Autodesk Inventor part; units mm, degrees
ref_plane "YZ Plane" through (0, 0, 0) normal (1, 0, 0) x (0, 1, 0)
ref_plane "XZ Plane" through (0, 0, 0) normal (0, 1, 0) x (-1, 0, 0)
ref_plane "XY Plane" through (0, 0, 0) normal (0, 0, 1) x (1, 0, 0)
sketch "Sketch1" plane through (0, 0, 0) normal (1, 0, 0) x (0, 1, 0)
  line L0 (0, 0) -> (12.5, 0)
  line L1 (12.5, 0) -> (12.5, -5)
  line L2 (12.5, -5) -> (0, -5)
  line L3 (0, 0) -> (0, 5)
  line L4 (0, 5) -> (15, 5)
  line L5 (15, 5) -> (15, -10)
  line L6 (15, -10) -> (0, -10)
  line L7 (0, -10) -> (0, -5)
  dimension "d0" = 12.5
  dimension "d2" = 5
  dimension "d3" = 15
  dimension "d4" = 15
  dimension "d5" = 5
extrude "Extrusion1" add sketch "Sketch1" along normal blind 27.5
sketch "Sketch2" plane through (0, 0, 5) normal (0, 0, 1) x (1, 0, 0)
  line L0 (0, 15) -> (27.5, 15)
  line L1 (0, 15) -> (0, 36)
  line L2 (0, 36) -> (2.5, 36)
  line L3 (0, 15) -> (39.5, 15)
  line L4 (39.5, 15) -> (39.5, 36)
  line L5 (39.5, 36) -> (37, 36)
  line L6 (37, 36) -> (37, 17.5)
  line L7 (37, 17.5) -> (2.5, 17.5)
  line L8 (2.5, 17.5) -> (2.5, 36)
  line L9 (0, 0) -> (27.5, 0)
  dimension "d8" = 21
  dimension "d9" = 2.5
  dimension "d10" = 39.5
  dimension "d11" = 2.5
  dimension "d12" = 18.5
  dimension "d13" = 17.5
extrude "Extrusion2" add sketch "Sketch2" against normal up to surface (15 mm away)
sketch "Sketch3" plane through (27.5, 0, -10) normal (0, 0, -1) x (-1, 0, 0)
  line L0 (27.5, 0) -> (22, 0)
  line L1 (22, 0) -> (22, 15)
  line L2 (22, 15) -> (27.5, 15)
  line L3 (27.5, 15) -> (27.5, 0)
  dimension "d16" = 5.5
  dimension "d17" = 15
extrude "Extrusion3" cut sketch "Sketch3" against normal up to surface (15 mm away)
sketch "Sketch4" plane through (37, 17.5, -10) normal (0, 0, -1) x (-1, 0, 0)
  line L0 (-2.5, -2.5) -> (9.5, -2.5)
  line L1 (37, 18.5) -> (34.5, 18.5)
  line L2 (-2.5, -2.5) -> (37, -2.5)
  line L3 (37, -2.5) -> (37, 18.5)
  line L4 (37, 18.5) -> (-2.5, 18.5)
  line L5 (-2.5, 18.5) -> (-2.5, -2.5)
  point P0 (37, -17.5)
extrude "Extrusion4" add sketch "Sketch4" along normal blind 2.5
sketch "Sketch5" plane through (2.5, 17.5, 5) normal (0, 0, 1) x (1, 0, 0)
  line L0 (37, -2.5) -> (25, -2.5)
  line L1 (37, 18.5) -> (37, -2.5)
  line L2 (34.5, 18.5) -> (37, 18.5)
  line L3 (34.5, 0) -> (34.5, 18.5)
  line L4 (0, 0) -> (34.5, 0)
  line L5 (0, 18.5) -> (0, 0)
  line L6 (-2.5, 18.5) -> (0, 18.5)
  line L7 (-2.5, -2.5) -> (-2.5, 18.5)
  line L8 (-2.5, -2.5) -> (3, -2.5)
  line L9 (37, 18.5) -> (37, -2.5)
  line L10 (37, -2.5) -> (25, -2.5)
  line L11 (37, 18.5) -> (34.5, 18.5)
  line L12 (34.5, 18.5) -> (34.5, 0)
  line L13 (34.5, -2.5) -> (37, -2.5)
  line L14 (37, -2.5) -> (37, 18.5)
  line L15 (0, 18.5) -> (0, 0)
  line L16 (-2.5, -2.5) -> (3, -2.5)
  line L17 (0, 18.5) -> (-2.5, 18.5)
  line L18 (-2.5, 18.5) -> (-2.5, -2.5)
  line L19 (-2.5, -2.5) -> (0, -2.5)
  line L20 (0, 0) -> (0, 18.5)
  line L21 (0, 0) -> (34.5, 0)
  line L22 (0, 0) -> (34.5, 0)
  line L23 (0, -2.5) -> (34.5, -2.5)
  line L24 (37, -2.5) -> (-2.5, -2.5)
  dimension "d22" = 34.5
  dimension "d23" = 34.5
extrude "Extrusion5" add sketch "Sketch5" along normal blind 2.5
sketch "Sketch6" plane through (2.5, 36, -10) normal (0, 1, 0) x (1, 0, 0)
  line L0 (37, -17.5) -> (37, 2.5)
  line L1 (-2.5, 2.5) -> (-2.5, -17.5)
  line L2 (37, 2.5) -> (-2.5, 2.5)
  line L3 (-2.5, 2.5) -> (-2.5, -17.5)
  line L4 (-2.5, -17.5) -> (37, -17.5)
  line L5 (37, -17.5) -> (37, 2.5)
  point P0 (-2.5, -10)
extrude "Extrusion6" add sketch "Sketch6" along normal blind 2.5
sketch "Sketch7" plane through (2.5, 17.5, 7.5) normal (0, 0, 1) x (1, 0, 0)
  line L0 (34.5, 18.5) -> (34.5, 0)
  line L1 (34.5, 0) -> (0, 0)
  line L2 (0, 0) -> (0, 18.5)
  line L3 (0, 18.5) -> (34.5, 18.5)
  line L4 (37, -2.5) -> (37, 21)
  line L5 (-2.5, 21) -> (37, 21)
  line L6 (-2.5, -2.5) -> (-2.5, 21)
  line L7 (-2.5, -2.5) -> (37, -2.5)
  line L8 (-2.5, -2.5) -> (37, -2.5)
  line L9 (37, 21) -> (34.5, 21)
  line L10 (34.5, 21) -> (34.5, -2.5)
  line L11 (34.5, -2.5) -> (37, -2.5)
  line L12 (37, -2.5) -> (37, 21)
  point P0 (-2.5, -17.5)
  dimension "d28" = 2.5
extrude "Extrusion7" cut sketch "Sketch7" against normal up to next contours L10 L5 L4 L7 L0
sketch "Sketch8" plane through (2.5, 17.5, 7.5) normal (0, 0, 1) x (1, 0, 0)
  line L0 (34.5, -2.5) -> (34.5, 0)
  line L1 (34.5, 0) -> (0, 0)
  line L2 (0, 0) -> (0, 18.5)
  line L3 (0, 18.5) -> (34.5, 18.5)
  line L4 (34.5, 18.5) -> (34.5, 21)
  line L5 (-2.5, 21) -> (34.5, 21)
  line L6 (-2.5, -2.5) -> (-2.5, 21)
  line L7 (-2.5, -2.5) -> (34.5, -2.5)
  line L8 (34.5, -2.5) -> (-2.5, -2.5)
  line L9 (-2.5, -2.5) -> (-2.5, 0)
  line L10 (0, 0) -> (34.5, 0)
  line L11 (34.5, 0) -> (34.5, -2.5)
  line L12 (34.5, 21) -> (-2.5, 21)
  line L13 (-2.5, 21) -> (-2.5, 18.5)
  line L14 (0, 18.5) -> (34.5, 18.5)
  line L15 (34.5, 18.5) -> (34.5, 21)
  line L16 (0, 18.5) -> (0, 0)
  line L17 (-2.5, 18.5) -> (-2.5, 0)
  dimension "d31" = 18.5
extrude "Extrusion8" add sketch "Sketch8" along normal blind 5
properties part number "battery-holder"
Can you work these out from the model? Positions are in its coordinate system, mm. A direction names the side the tool comes from. Coordinates: 2 decimals unless noted, no trailing zeros. Loops run counter-clockwise (first coordinate to the right, second up) from the corner with the lowest first, then second, coordinate; pieces in that order, holes last. Notation, with made-up numbers: (46.25, 62.25) - (60.25, 62.25) arc R12 cw to (60.25, 78.25) - close; hole circle Ø7 at (52, 85). An arc over 180 degrees is marked (long way). Answer as a JSON object with one key per item and string values. Group by question number.
Item 1: If we section it at A-A (y = 6.5): List the corners of the cut face in (x, z) for me, plus the area to 3 significant figures.
Item 2: If we section it at C-C (z = -7.75): List the corners of the cut face in (x, y) for me, plus the area to 3 significant figures.
Item 3: For pin 1 (6 mm diameter, centred on x = 25.5, z = -6, fed in from -Y); pin 2 (4.5 mm diameter, centred on x = 17, y = 4.5, fed in from +Z); pin 3 (1.5 mm diameter, centred on y = 23, z = -8, fed in from +X); pin 4 (6 mm diameter, centred on x = 21, y = 9, fed in from -Z), each with a flat end and sliding along its axis, tell me the tip position at first contact or that it passes through.
Item 4: If I drill on L1, parallel to Y at x = 26, z = -2; L2, parallel to Z at x = 18.5, y = 2; L3, parallel to Y at x = 6, z = 11.25, over which ranges is the centre line in solid material (lowest first)? Write a range as from..to.
Item 5: If we section it at D-D (y = 33): List the corners of the cut face in (x, z) for me.
Item 6: If we section it at B-B (x = 9.5): List the corners of the cut face in (y, z) for me, plus the area to 3 significant figures.
Item 7: On a 3-axis mill with a long thin cutter (end or side, diameter ignored), from which of +Z, -Z, +X, -X, +Y, -Y can I reach the whole of each face in a straight line? I mean faces 4 (the face through (16, 8, -10)), 5 (the face through (16, 6, -5)), 6 (the face through (5.5, 7, 1)), 7 (the face through (2.5, 27, 1)). Say none if no direction works.
Item 8: If we mould it in two halves opening along Z, with no side actions, what happens to faces 1 (the face through (16, 7, 5)), 2 (the face through (16, 6, 0)), 3 (the face through (20, 17.5, 1))? For each: released by +Z, released by -Z, zero draft, split by the parting line, or undercut.
Returned:
{
 "1": {"outline": "(5.5, -10) - (27.5, -10) - (27.5, -5) - (5.5, -5) - close; (5.5, 0) - (27.5, 0) - (27.5, 5) - (5.5, 5) - close", "area": "220 mm²"},
 "2": {"outline": "(0, 15) - (5.5, 15) - (5.5, 0) - (27.5, 0) - (27.5, 15) - (37, 15) - (37, 17.5) - (2.5, 17.5) - (2.5, 36) - (37, 36) - (37, 38.5) - (0, 38.5) - close", "area": "561 mm²"},
 "3": {"pin 1": "stops at y = 0", "pin 2": "stops at z = 5", "pin 3": "stops at x = 2.5", "pin 4": "stops at z = -10"},
 "4": {"L1": "y = 12.5..17.5, 36..38.5", "L2": "z = -10..-5, 0..5", "L3": "y = 15..17.5, 36..38.5"},
 "5": {"outline": "(0, -12.5) - (37, -12.5) - (37, -10) - (2.5, -10) - (2.5, 12.5) - (0, 12.5) - close"},
 "6": {"outline": "(0, -10) - (15, -10) - (15, -12.5) - (38.5, -12.5) - (38.5, 12.5) - (36, 12.5) - (36, -10) - (17.5, -10) - (17.5, 12.5) - (15, 12.5) - (15, 5) - (0, 5) - (0, 0) - (12.5, 0) - (12.5, -5) - (0, -5) - close", "area": "334 mm²"},
 "7": {"face 4": "-Z, +X, -X, -Y", "face 5": "+X, -X, -Y", "face 6": "+Z, -Z, -X, -Y", "face 7": "+Z, +X"},
 "8": {"face 1": "released by +Z", "face 2": "undercut", "face 3": "zero draft"}
}
